from build123d import *

# Parameters (mm, degrees)
F0_W      = 3
F0_H      = 5
F1_DEPTH  = 10
F2_R      = 1
F4_COUNT  = 3
F4_ANGLE  = 240
F5_R      = 7.5
F6_DEPTH  = 11
F9_D      = 1
F9_DEPTH  = 1
F9_TIP    = 0.3004303095
F10_D     = 6
F10_DEPTH = 1
F10_TIP   = 1.8025818571


with BuildPart() as f1:
    # F0 (on Top) → F1 (new body)
    with BuildSketch(Plane.XY):
        with Locations((0, 0.5)):
            Rectangle(F0_W, F0_H)
    extrude(amount=F1_DEPTH)

    # F2
    f2_edges = [f1.edges().sort_by_distance(p)[0] for p in [
        (-1.5, 3, 5),
        (1.5, 3, 5),
    ]]
    fillet(f2_edges, radius=F2_R)

    # F4: F1 ×3 about axis
    f4_axis = Axis((0, 0, 4.9742138945), (0, 0, -1))


with BuildPart() as f1_1:
    add(f1.part)
    for i in range(1, F4_COUNT):
        add(f1.part.rotate(f4_axis, i * F4_ANGLE / (F4_COUNT - 1)))


with BuildPart() as f6:
    # F5 (on Top) → F6 (new body)
    with BuildSketch(Plane.XY):
        Circle(F5_R)
    extrude(amount=F6_DEPTH)

    # F7: cut F1
    add(f1_1.part, mode=Mode.SUBTRACT)

    # F9
    with Locations(Plane.XY.offset(11)):
        with Locations((-6, 0), (6, 0), (0, 6), (0, -6)):
            Hole(F9_D / 2, depth=F9_DEPTH)
            with Locations((0, 0, -(F9_DEPTH + F9_TIP / 2))):  # 118° drill point
                Cone(0, F9_D / 2, F9_TIP, mode=Mode.SUBTRACT)

    # F10
    with Locations(Plane.XY.offset(11)):
        with Locations((0, 0)):
            Hole(F10_D / 2, depth=F10_DEPTH)
            with Locations((0, 0, -(F10_DEPTH + F10_TIP / 2))):  # 118° drill point
                Cone(0, F10_D / 2, F10_TIP, mode=Mode.SUBTRACT)


solid = f6.part
The model under review builds one solid part; all positions refer to its coordinate system, in mm. A direction names the side the tool comes from. Give positions to 0.01 mm unless a question says otherwise; leave off trailing zeros. Loops run counter-clockwise (first coordinate to the right, second up) from the corner with the lowest first, then second, coordinate; pieces in that order, holes last. Notation, with made-up numbers: (-5.5, 24.25) -> (10.5, 24.25) arc R21 ccw to (10.5, 36.25) -> close; hole circle Ø11 at (38.25, 80.5). An arc over 180 degrees is marked (long way). Put each result on its own line as item: value. Start each with the question number.
1. Mouldability with a two-part tool opening along X and no side actions: class faces 4 (the face through (3.2, 0.1, 11)), 5 (the face through (1.73, -2.4, 5.07)) as released by +X, released by -X, zero draft, split by the parting line, or undercut.
2. Wall thickness on probe 1 along Y at (x, z) = (0, 10.2); probe 2 along X at (y, z) = (-3.75, 7); probe 3 along Y at (x, z) = (-6, 10.4): over which ranges is each line inside the solid? List them lowest first.
3. Clearance check with flat-ended pins moving along their axes: P1, Ø0.7, axis at y = 1.5, z = 3.5, coming from the -X side; P2, Ø5, axis at x = -2.5, z = 3, coming from the -Y side; P3, Ø3, axis at y = -3, z = 8, coming from the +X side. State where each tip first meets the part, or that it passes through.
4. We need section C-C on y = 3.5. State the section outline as (x, z) points.
5. For faces 1 (the face through (0, -2.5, 9.7)), 2 (the face through (0, -2, 5)), 3 (the face through (0, 3, 5)), list the 3-axis set-ups (+Z, -Z, +X, -X, +Y, -Y) from which the entire face can be reached by the end or side of a thin tool; tool diameter is ignored.
6. We need section A-A on z = 8.5. State the section outline as (x, y) points.
7. We need section B-B on x = -4. State the section outline as (y, z) points, then the cut area to 3 significant figures.
Determined:
1. face 4: zero draft
1. face 5: undercut
2. probe 1: -7.5 to -6.5, -5.5 to -3, 3 to 5.5, 6.5 to 7.5
2. probe 2: -6.5 to 6.5
2. probe 3: -4.5 to -0.5, 0.5 to 4.5
3. P1: x = -7.41
3. P2: y = -7.5
3. P3: x = 7.35
4. outline: (-6.63, 0) -> (6.63, 0) -> (6.63, 11) -> (-6.63, 11) -> close
5. face 1: +Z
5. face 2: +Z, -Z
5. face 3: -Z
6. outline: circle Ø15 at (0, 0); hole (-2.85, -1.07) -> (-2.35, -1.93) arc R1 ccw to (-0.98, -2.3) -> (-0.46, -2) -> (0.46, -2) -> (0.98, -2.3) arc R1 ccw to (2.35, -1.93) -> (2.85, -1.07) arc R1 ccw to (2.48, 0.3) -> (1.96, 0.6) -> (1.5, 1.4) -> (1.5, 2) arc R1 ccw to (0.5, 3) -> (-0.5, 3) arc R1 ccw to (-1.5, 2) -> (-1.5, 1.4) -> (-1.96, 0.6) -> (-2.48, 0.3) arc R1 ccw to start
7. outline: (-6.34, 0) -> (6.34, 0) -> (6.34, 11) -> (-6.34, 11) -> close
7. area: 140 mm^2
